Drawing for the job (mm, zero at the part's lowest x, y, z). Round coordinates to 2 decimals unless told otherwise and drop trailing zeros. Write each loop counter-clockwise with the first axis right and the second up, starting at its lowest first coordinate (ties: lowest second). Pieces come first, ordered by that corner, then holes.
Item 1: Wall check: probe 1 along Y at (x, z) = (4, 11); probe 2 along Y at (x, z) = (5.75, 7.5); probe 3 along X at (y, z) = (5.5, 13.5). Give the ranges that are in metal, low to high.
Item 2: Mould opens along X. For the marked faces 1, 2 and 3 say: +X half, -X half, draft (parallel to the pull), parting line (faces both ways), or undercut.
Item 3: Band-saw the part on C-C, the plane z = 1.75. Write the cut outline in (x, y), then the cut area to 3 significant figures.
Item 4: Band-saw the part on A-A, the plane y = 4. Write the cut outline in (x, z).
Item 5: Drop a flat-ended pin along its axis: pin 1 Ø2 at (y, z) = (6, 7) entering from -X. Give the stop position or say it passes through.
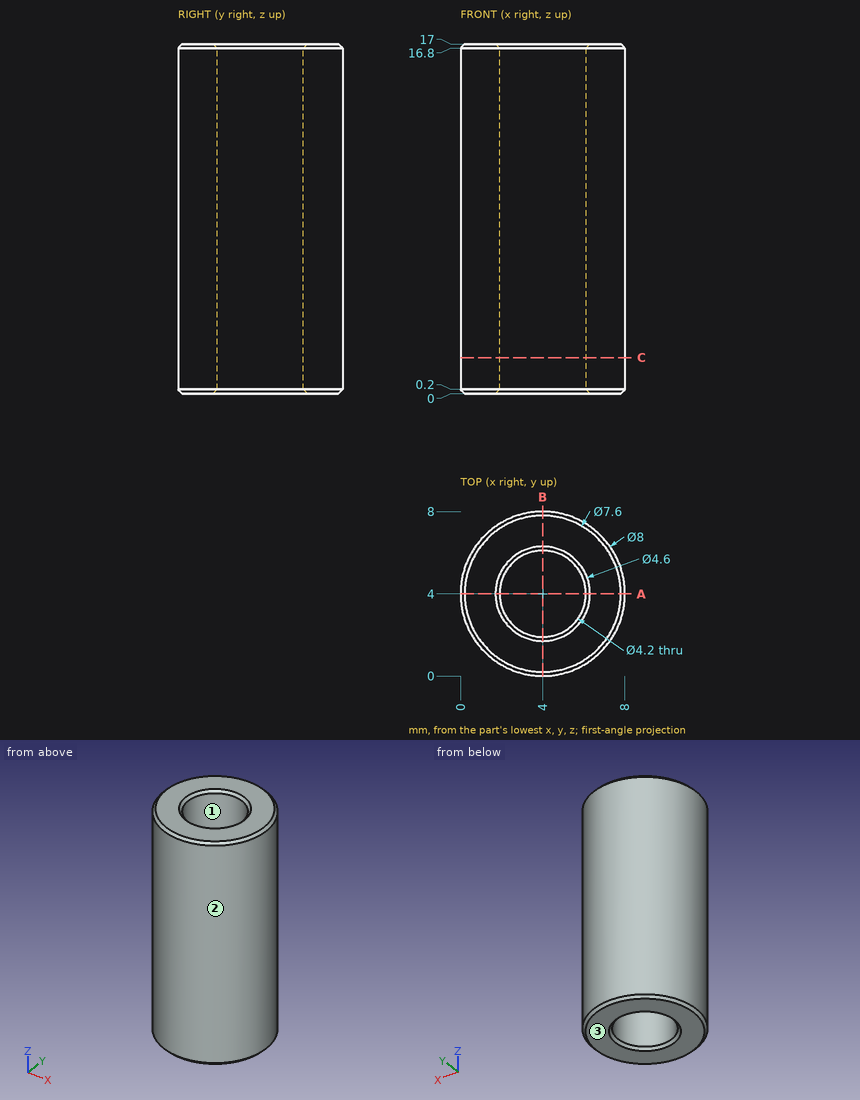
Results:
1. probe 1: y = 0 to 1.9, 6.1 to 8
1. probe 2: y = 0.4 to 2.84, 5.16 to 7.6
1. probe 3: x = 0.29 to 2.53, 5.47 to 7.71
2. face 1: undercut
2. face 2: parting line
2. face 3: draft
3. outline: circle Ø8 at (4, 4); hole circle Ø4.2 at (4, 4)
3. area: 36.4 mm2
4. outline: (0, 0.2) - (0.2, 0) - (1.7, 0) - (1.9, 0.2) - (1.9, 16.8) - (1.7, 17) - (0.2, 17) - (0, 16.8) - close; (6.1, 0.2) - (6.3, 0) - (7.8, 0) - (8, 0.2) - (8, 16.8) - (7.8, 17) - (6.3, 17) - (6.1, 16.8) - close
5. pin 1: stops at x = 0.13
